Here's how the part is built. I have some questions about the finished solid (model axes, mm). A direction names the side the tool comes from. Round coordinates to 2 decimals unless told otherwise and drop trailing zeros. Write each loop counter-clockwise with the first axis right and the second up, starting at its lowest first coordinate (ties: lowest second). Pieces come first, ordered by that corner, then holes. Notation, with made-up numbers: (3, 55) -> (47, 55) arc R36 ccw to (47, 94) -> close; hole circle Ø6 at (72, 76.5). An arc over 180 degrees is marked (long way). Put each result on its own line as item: value. Start each with the question number.
1. Suppose I cut it at A-A (z = 2.05). Please give me the cut outline in (x, y).
2. We'd pull the mould along X, two halves only. Please class faces 6 (the face through (10, 8, 1)), 7 (the face through (0, 0, 0)), 8 (the face through (20, 0, 1)): +X half, -X half, draft (parallel to the pull), parting line (faces both ways), or undercut.
3. For pin 1 (0.9 mm diameter, centred on y = 8.5, z = 1, fed in from -X); pin 2 (1.5 mm diameter, centred on x = 18, z = 2, fed in from +Y), each with a flat end and sliding along its axis, tell me the tip position at first contact or that it passes through.
4. Which directions (+Z, -Z, +X, -X, +Y, -Y) give clear straight access to the entire face, cutting with the end or side of a thin tool? Please do faces 1 (the face through (0, 0, 3)), 2 (the face through (-13, 9.65, 1)), 3 (the face through (18, 6.65, 1)), 4 (the face through (-10, 8, 1)), 5 (the face through (-16, 8, 1)).
5. I need wall thicknesses on probe 1 along Y at (x, z) = (6, 0.45). Which ranges of the line are inside material? Lowest first, please. Write a range as from..to.
6. Suppose I cut it at B-B (x = 7). Please give me the cut outline in (y, z), then the cut area to 3 significant figures.
```python
from build123d import *

# Parameters (mm, degrees)
SKETCH1_W           = 6
SKETCH1_H           = 3
BOSS_EXTRUDE1_DEPTH = 3


with BuildPart() as part:
    # Sketch1 → Boss-Extrude1 (new body)
    with BuildSketch(Plane.XY):
        Polygon((0, -6.65), (0, 6.65), (-10, 6.65), (-16, 6.65), (-20, 6.65), (-20, -6.65), align=None)
        Polygon((10, 6.65), (0, 6.65), (0, -6.65), (20, -6.65), (20, 6.65), (16, 6.65), align=None)
        with Locations((13, 8.15)):
            Rectangle(SKETCH1_W, SKETCH1_H)
        with Locations((-13, 8.15)):
            Rectangle(SKETCH1_W, SKETCH1_H)
    extrude(amount=BOSS_EXTRUDE1_DEPTH)


solid = part.part
```
Verdict:
1. outline: (-20, -6.65) -> (20, -6.65) -> (20, 6.65) -> (16, 6.65) -> (16, 9.65) -> (10, 9.65) -> (10, 6.65) -> (-10, 6.65) -> (-10, 9.65) -> (-16, 9.65) -> (-16, 6.65) -> (-20, 6.65) -> close
2. face 6: undercut
2. face 7: draft
2. face 8: +X half
3. pin 1: stops at x = -16
3. pin 2: stops at y = 6.65
4. face 1: +Z, +X, -X, +Y, -Y
4. face 2: +Z, -Z, +X, -X, +Y
4. face 3: +Z, -Z, +X, +Y
4. face 4: +Z, -Z, +Y
4. face 5: +Z, -Z, -X, +Y
5. probe 1: y = -6.65..6.65
6. outline: (-6.65, 0) -> (6.65, 0) -> (6.65, 3) -> (-6.65, 3) -> close
6. area: 39.9 mm^2
